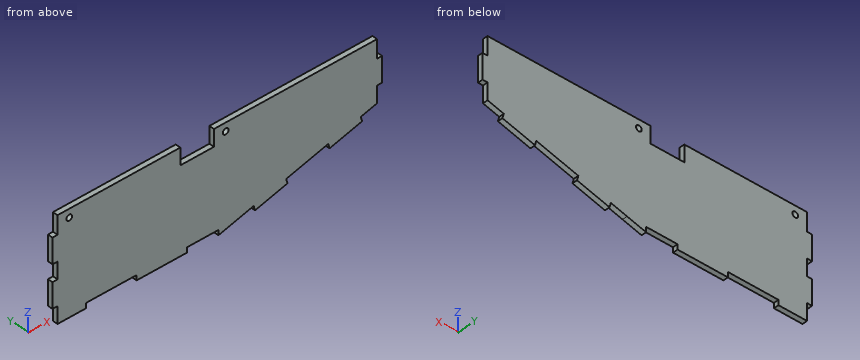
from build123d import *

# Parameters (mm, degrees)
SKETCH1_W           = 196
SKETCH1_H           = 61
BOSS_EXTRUDE1_DEPTH = 3
SKETCH2_R           = 1.7
SKETCH2_W           = 3
SKETCH2_H           = 10
SKETCH2_H_2         = 11
SKETCH2_W_2         = 30
SKETCH2_H_3         = 3
SKETCH2_W_3         = 20
CUT_EXTRUDE1_DEPTH  = 3
CUT_EXTRUDE2_DEPTH  = 10
BOSS_EXTRUDE2_DEPTH = 3


with BuildPart() as part:
    # Sketch1 → Boss-Extrude1 (new body)
    with BuildSketch(Plane(origin=(0, 0, 0), x_dir=(1, 0, 0), z_dir=(0, 1, 0))):
        Rectangle(SKETCH1_W, SKETCH1_H)
    extrude(amount=BOSS_EXTRUDE1_DEPTH)

    # Sketch2 → Cut-Extrude1 (cut)
    with BuildSketch(Plane(origin=(0, 3, 0), x_dir=(1, 0, 0), z_dir=(0, 1, 0))):
        with Locations(Location((-88, -25.5, 0), (0, 0, 270))):
            Circle(SKETCH2_R)
        with Locations(Location((5, -25.5, 0), (0, 0, 270))):
            Circle(SKETCH2_R)
        with Locations((-96.5, 25.5)):
            Rectangle(SKETCH2_W, SKETCH2_H)
        with Locations((-96.5, 0.5)):
            Rectangle(SKETCH2_W, SKETCH2_H)
        with Locations((-96.5, -25)):
            Rectangle(SKETCH2_W, SKETCH2_H_2)
        with Locations((96.5, 0.5)):
            Rectangle(SKETCH2_W, SKETCH2_H)
        with Locations((96.5, -25)):
            Rectangle(SKETCH2_W, SKETCH2_H_2)
        with Locations((57, 29)):
            Rectangle(SKETCH2_W_2, SKETCH2_H_3)
        with Locations((-12, -25.5)):
            Rectangle(SKETCH2_W_3, SKETCH2_H)
        with Locations((-63, 29)):
            Rectangle(SKETCH2_W_2, SKETCH2_H_3)
        with Locations((-3, 29)):
            Rectangle(SKETCH2_W_2, SKETCH2_H_3)
        with Locations((96.5, 25.5)):
            Rectangle(SKETCH2_W, SKETCH2_H)
    extrude(amount=-CUT_EXTRUDE1_DEPTH, mode=Mode.SUBTRACT)

    # Sketch3 → Cut-Extrude2 (cut)
    with BuildSketch(Plane(origin=(0, 3, 0), x_dir=(1, 0, 0), z_dir=(0, 1, 0))):
        Polygon((12, 30.5), (98, 30.5), (98, 5.5), (95, 5.5), (85.333795578, 8.062126473), (86.10243352, 10.9619878), (66.770024675, 16.086240747), (66.001386733, 13.18637942), (40.998613267, 19.81362058), (41.767251209, 22.713481907), (22.434842364, 27.837734853), (21.666204422, 24.937873527), (12, 27.5), align=None)
    extrude(amount=-CUT_EXTRUDE2_DEPTH, mode=Mode.SUBTRACT)

    # Sketch4 → Boss-Extrude2 (add)
    with BuildSketch(Plane(origin=(0, 3, 0), x_dir=(1, 0, 0), z_dir=(0, 1, 0))):
        Polygon((12, 27.5), (0.681818182, 30.5), (0.681818182, 27.5), align=None)
    extrude(amount=-BOSS_EXTRUDE2_DEPTH)


solid = part.part
Could you check a few things on this model? Use its own coordinates, in mm. Give positions to 0.01 mm unless a question says otherwise; leave off trailing zeros. Order: outer loops, then holes, each group sorted by start corner. A loop starts at its lowest first (then second) coordinate and runs counter-clockwise, first axis right, second up. Notation, with made-up numbers: (67.5, 75) -> (119.5, 75) arc R15 cw to (119.5, 99) -> close; hole circle Ø5 at (35.25, 20.5). An arc over 180 degrees is marked (long way). Return JSON: item names as keys, results as strings.
1. Imagine slicing it at C-C on y = 1.25. Give the number of separate pieces and of enclosed holes in the cut face, then the cut area to 3 significant figures.
Answer list:
{"separate pieces": "1", "enclosed holes": "2", "area": "10,300 mm2"}
2. Imagine slicing it at B-B on z = 25.5. List the corners of the cut face in (x, y) for me, then the cut area to 3 significant figures.
Answer list:
{"outline": "(-95, 0) -> (-89.7, 0) -> (-89.7, 3) -> (-95, 3) -> close; (-86.3, 0) -> (-22, 0) -> (-22, 3) -> (-86.3, 3) -> close; (-2, 0) -> (3.3, 0) -> (3.3, 3) -> (-2, 3) -> close; (6.7, 0) -> (95, 0) -> (95, 3) -> (6.7, 3) -> close", "area": "490 mm2"}
3. For pin 1 Ø1.5 at (y, z) = (1.5, -28) entering from -X; pin 2 Ø0.9 at (y, z) = (1, 25) entering from +X; pin 3 Ø1.5 at (x, y) = (-96.5, 1.5) entering from -Z; pin 4 Ø12 at (x, z) = (-74.5, -9.5) entering from -Y, each with a flat end and sliding along its axis, tell me the tip position at first contact or that it passes through.
Answer list:
{"pin 1": "stops at x = -95", "pin 2": "stops at x = 95", "pin 3": "stops at z = -20.5", "pin 4": "stops at y = 0"}
4. I need wall thicknesses on line 1 (X direction, y = 1, z = 25.5); line 2 (Z direction, x = -88, y = 0.8); line 3 (X direction, y = 1.6, z = -4.5). Which ranges of each line are inside material? Lowest first, please. Write a range as from..to.
Answer list:
{"line 1": "x = -95..-89.7, -86.3..-22, -2..3.3, 6.7..95", "line 2": "z = -30.5..23.8, 27.2..30.5", "line 3": "x = -95..95"}
5. Imagine slicing it at D-D on x = 5. List the corners of the cut face in (y, z) for me, then the cut area to 3 significant figures.
Answer list:
{"outline": "(0, -29.36) -> (3, -29.36) -> (3, 23.8) -> (0, 23.8) -> close; (0, 27.2) -> (3, 27.2) -> (3, 30.5) -> (0, 30.5) -> close", "area": "169 mm2"}
6. Imagine slicing it at A-A on x = -88. List the corners of the cut face in (y, z) for me.
Answer list:
{"outline": "(0, -30.5) -> (3, -30.5) -> (3, 23.8) -> (0, 23.8) -> close; (0, 27.2) -> (3, 27.2) -> (3, 30.5) -> (0, 30.5) -> close"}
